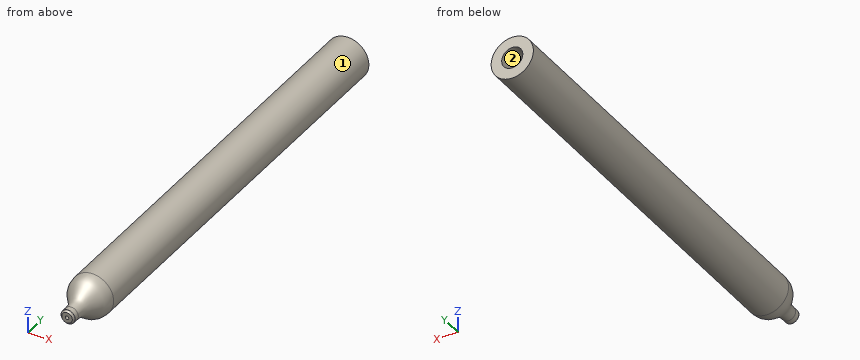
from build123d import *

# Parameters (mm, degrees)
CHAMFER1_SIZE = 0.25
FILLET1_R     = 0.1


with BuildPart() as part:
    # Sketch1 → Revolve1 (revolve)
    with BuildSketch(Plane.XY):
        with BuildLine():
            Line((1.5, 61), (3, 61))
            Line((3, 61), (3, 1))
            add(Edge.make_bspline(
                [(1, -4), (1, -2.852326224), (1, -1.704652447), (3, -1.295347553), (3, -0.147673776), (3, 1)],
                knots=[0, 0, 0, 0, 0, 0, 1, 1, 1, 1, 1, 1], degree=5))
            Line((1, -4), (1, -5))
            Line((1, -5), (0.25, -5))
            Line((0.25, -5), (0.25, -4))
            add(Edge.make_bspline(
                [(0.25, -4), (0.25, -3.874328316), (0.348, -1.569029575), (1.407157895, -1.561541747), (1.5, -0.081983242), (1.5, 0)],
                knots=[0, 0, 0, 0, 0.05, 0.95, 1, 1, 1, 1], degree=3))
            Line((1.5, 0), (1.5, 61))
        make_face()
    revolve(axis=Axis((0, 0, 0), (0, -1, 0)))

    # Chamfer1
    chamfer1_edges = [part.edges().sort_by_distance(p)[0] for p in [
        (-1, -5, 0),
    ]]
    chamfer(chamfer1_edges, length=CHAMFER1_SIZE)

    # Fillet1
    fillet1_edges = [part.edges().sort_by_distance(p)[0] for p in [
        (-1, -4.75, 0),
    ]]
    fillet(fillet1_edges, radius=FILLET1_R)


solid = part.part
Here's how the part is built. I have some questions about the finished solid (model axes, mm). Face numbers are marked on the shaded views. Coordinates: 2 decimals unless noted, no trailing zeros. Write each loop counter-clockwise with the first axis right and the second up, starting at its lowest first coordinate (ties: lowest second). Pieces come first, ordered by that corner, then holes.
1) If I drill on line 1 (Z direction, x = 0, y = -4.5); line 2 (X direction, y = 16, z = -0.5); line 3 (Z direction, x = 0, y = 47), over which ranges is the centre line in solid material (lowest first)?
Filled in:
line 1: z = -1 to -0.25, 0.25 to 1
line 2: x = -2.96 to -1.41, 1.41 to 2.96
line 3: z = -3 to -1.5, 1.5 to 3
2) I'm going to push flat-ended pins straight in: pin 1 (1.5 mm diameter, centred on x = 2, y = 13.5, fed in from -Z); pin 2 (1 mm diameter, centred on y = 16.5, z = -1, fed in from -X); pin 3 (2 mm diameter, centred on x = 2.5, z = -0.5, fed in from -Y). Where does each tip first touch, or does it pass through?
Filled in:
pin 1: stops at z = -2.73
pin 2: stops at x = -2.96
pin 3: stops at y = -2.05
3) Thinking about a two-plate mould opening in Z: for the marked faces 1 and 2, which applies, +Z half, -Z half, draft (parallel to the pull), parting line (faces both ways), or undercut?
Filled in:
face 1: parting line
face 2: undercut
4) If we section it at A-A (y = 32.5): List the corners of the cut face in (x, z) for me.
Filled in:
outline: circle Ø6 at (0, 0); hole circle Ø3 at (0, 0)
